```python
from build123d import *

# Parameters (mm, degrees)
REVOLVE_1_ANGLE     = 180
FILLET_1_R          = 5
FILLET_2_R          = 5
SKETCH_2_W          = 12
SKETCH_2_H          = 5
CUT_EXTRUDE_1_DEPTH = 6


with BuildPart() as part:
    # 草图1 → 旋转1 (revolve)
    with BuildSketch(Plane.XY):
        with BuildLine():
            Line((-15, 5), (15, 5))
            ThreePointArc((15, 5), (14.412847263, 11.739422714), (12.669081334, 18.275770872))
            ThreePointArc((12.669081334, 18.275770872), (0, 20), (-12.669081334, 18.275770872))
            ThreePointArc((-12.669081334, 18.275770872), (-14.412847263, 11.739422714), (-15, 5))
        make_face()
    revolve(axis=Axis((-17.5, 0, 0), (1, 0, 0)), revolution_arc=REVOLVE_1_ANGLE)

    # 圆角1
    fillet_1_edges = [part.edges().sort_by_distance(p)[0] for p in [
        (12.669081334, 0, 18.275770872),
        (-12.669081334, 0, 18.275770872),
    ]]
    fillet(fillet_1_edges, radius=FILLET_1_R)

    # 圆角2
    fillet_2_edges = [part.edges().sort_by_distance(p)[0] for p in [
        (-15, 0, 5),
        (15, 0, 5),
    ]]
    fillet(fillet_2_edges, radius=FILLET_2_R)

    # 草图2 → 切除-拉伸1 (cut)
    with BuildSketch(Plane(origin=(0, 0, 0), x_dir=(-1, 0, 0), z_dir=(0, 0, -1))):
        with Locations((0, 12)):
            Rectangle(SKETCH_2_W, SKETCH_2_H)
        with Locations((0, -12)):
            Rectangle(SKETCH_2_W, SKETCH_2_H)
    extrude(amount=-CUT_EXTRUDE_1_DEPTH, mode=Mode.SUBTRACT)


solid = part.part
```
Work out the finished part from the listing and answer in its coordinate system (mm). A direction names the side the tool comes from. Coordinates: 2 decimals unless noted, no trailing zeros.
Q1. Each of these flat-tipped pins is pushed along its axis until it touches: pin 1 Ø1.5 at (x, y) = (-8.5, 16) entering from +Z; pin 2 Ø8 at (x, z) = (-4, 11.5) entering from +Y; pin 3 Ø1.8 at (x, z) = (1, 3) entering from +Y; pin 4 Ø1 at (y, z) = (-2.5, 3) entering from -X. Where does it stop, or does it pass through?
Q2. Which of the six approach directions +Z, -Z, +X, -X, +Y, -Y give full straight-line access (tool end or side, diameter ignored) to faces 3 (the face through (0, -9.5, 3)), 4 (the face through (0, 0, 5))?
Q3. Find the intervals of material crossed by line 1 (Y direction, x = -5.75, z = 1.5); line 2 (Y direction, x = -3.25, z = 4.25); line 3 (X direction, y = 6.5, z = 6.5), in increasing order.
Q4. Determine the mould class of faces 1 (the face through (0, 9, 0)), 2 (the face through (6, 12, 3)) for opening direction Y: released by +Y, released by -Y, zero draft, split by the parting line, or undercut.
Findings below:
1. pin 1: stops at z = 11.74
1. pin 2: stops at y = 18.39
1. pin 3: stops at y = 19.88
1. pin 4: passes through
2. face 3: -Z
2. face 4: -Z, +X, -X
3. line 1: y = -19.59 to -14.5, -9.5 to -4.77, 4.77 to 9.5, 14.5 to 19.59
3. line 2: y = -19.43 to -14.5, -9.5 to -2.63, 2.63 to 9.5, 14.5 to 19.43
3. line 3: x = -14.56 to 14.56
4. face 1: zero draft
4. face 2: undercut
